Design review of the part built by this model. Coordinates are the model's own, in mm. Give positions to 0.01 mm unless a question says otherwise; leave off trailing zeros. Write each loop counter-clockwise with the first axis right and the second up, starting at its lowest first coordinate (ties: lowest second). Pieces come first, ordered by that corner, then holes.
```python
from build123d import *

# Parameters (mm, degrees)
F0_W      = 177.8
F0_H      = 25.4
F1_DEPTH  = 2.54
F2_R      = 3.175
F3_DEPTH  = 25.4
F4_DEPTH  = 25.4
F5_DEPTH  = 127
F6_R      = 3.175
F7_DEPTH  = 25.4
F8_DEPTH  = 127
F9_R      = 3.175
F10_DEPTH = 25.4


with BuildPart() as f1:
    # F0 (on Front) → F1 (new body)
    with BuildSketch(Plane.XZ):
        Rectangle(F0_W, F0_H)
    extrude(amount=F1_DEPTH)

    # F2 (on Front) → F3 (join)
    with BuildSketch(Plane.XZ):
        with Locations((-31.75, 0)):
            Circle(F2_R)
        with Locations((31.75, 0)):
            Circle(F2_R)
    extrude(amount=F3_DEPTH)

    # F2 (on Front) → F4 (join)
    with BuildSketch(Plane.XZ):
        with Locations((-31.75, 0)):
            Circle(F2_R)
        with Locations((31.75, 0)):
            Circle(F2_R)
        with Locations((76.2, 0)):
            Circle(F2_R)
    extrude(amount=F4_DEPTH)

    # F5 (add): a face of the model
    f5_faces = [f1.faces().sort_by_distance(p)[0] for p in [
        (-88.9, -1.27, 0),
    ]]
    extrude(f5_faces, amount=F5_DEPTH)

    # F6 (on face) → F7 (join)
    with BuildSketch(Plane.XZ.offset(2.54)):
        with Locations((-184.15, 0)):
            Circle(F6_R)
    extrude(amount=F7_DEPTH)

    # F8 (add): a face of the model
    f8_faces = [f1.faces().sort_by_distance(p)[0] for p in [
        (88.9, -1.27, 0),
    ]]
    extrude(f8_faces, amount=F8_DEPTH)

    # F9 (on face) → F10 (join)
    with BuildSketch(Plane.XZ.offset(2.54)):
        with Locations((152.4, 0)):
            Circle(F9_R)
        with Locations((177.8, 0)):
            Circle(F9_R)
        with Locations((203.2, 0)):
            Circle(F9_R)
    extrude(amount=F10_DEPTH)


solid = f1.part
```
(1) Consider section C-C, the plane z = 7.5. Give the boundary of the cut face in (x, y).
Resolved:
outline: (-215.9, -2.54) - (215.9, -2.54) - (215.9, 0) - (-215.9, 0) - close
(2) Mouldability with a two-part tool opening along X and no side actions: class faces 1 (the face through (-3, -2.54, 0)), 2 (the face through (-3, 0, 0)) as pulls with the +X half, pulls with the -X half, needs draft (parallel to the pull), parting line crosses it, or undercut.
Resolved:
face 1: undercut
face 2: needs draft
(3) To check wall thickness, follow L1, parallel to Y at x = 166, z = 8.25; L2, parallel to X at y = -26.5, z = 2. State the ranges of each line that lie inside material, in increasing order.
Resolved:
L1: y = -2.54 to 0
L2: x = -186.62 to -181.68, 149.93 to 154.87, 175.33 to 180.27, 200.73 to 205.67
(4) Consider section A-A, the plane y = -7. Give the boundary of the cut face in (x, z) (3 decimals), then the cut area to 3 significant figures.
Resolved:
outline: circle Ø6.35 at (-184.15, 0); circle Ø6.35 at (-31.75, 0); circle Ø6.35 at (31.75, 0); circle Ø6.35 at (76.2, 0); circle Ø6.35 at (152.4, 0); circle Ø6.35 at (177.8, 0); circle Ø6.35 at (203.2, 0)
area: 222 mm2
(5) Consider section B-B, the plane x = 0. Give the boundary of the cut face in (y, z).
Resolved:
outline: (-2.54, -12.7) - (0, -12.7) - (0, 12.7) - (-2.54, 12.7) - close
(6) Clearance check with flat-ended pins moving along their axes: P1, Ø7.5, axis at x = 60.5, z = -5.5, coming from the -Y side; P2, Ø1, axis at y = -24, z = 3, coming from the +X side; P3, Ø5, axis at x = 32.5, z = 0.5, coming from the -Y side; P4, Ø10, axis at x = 60, z = 5, coming from the +Y side. State where each tip first meets the part, or that it passes through.
Resolved:
P1: stops at y = -2.54
P2: stops at x = 205.16
P3: stops at y = -25.4
P4: stops at y = 0
